For this review, take the finished solid that the model builds, in its own axes (mm). A direction names the side the tool comes from. Round coordinates to 2 decimals unless told otherwise and drop trailing zeros. Order: outer loops, then holes, each group sorted by start corner. A loop starts at its lowest first (then second) coordinate and runs counter-clockwise, first axis right, second up.
from build123d import *

# Parameters (mm, degrees)
EXTRUDE_1_DEPTH     = 28
SKETCH_2_W          = 5
SKETCH_2_H          = 20
CUT_EXTRUDE_1_DEPTH = 5
SKETCH_3_R          = 1.5
CUT_EXTRUDE_2_DEPTH = 118.553755913


with BuildPart() as part:
    # 草圖1 → 填料-伸長1 (new body)
    with BuildSketch(Plane.XY):
        Polygon((-17.451364004, -6.196122823), (-17.451364004, -11.196122823), (-22.451364004, -11.196122823), (-22.451364004, 105.303877177), (-17.451364004, 105.303877177), (-17.451364004, 100.303877177), (24.548635996, 100.303877177), (24.548635996, 95.303877177), (-17.451364004, 95.303877177), (-17.451364004, -1.196122823), (16.048635996, -1.196122823), (16.048635996, -6.196122823), align=None)
    extrude(amount=EXTRUDE_1_DEPTH)

    # 草圖2 → 除料-伸長1 (cut)
    with BuildSketch(Plane(origin=(0, 0, 0), x_dir=(-1, 0, 0), z_dir=(0, 0, -1))):
        with Locations((19.951364004, 47.053877177)):
            Rectangle(SKETCH_2_W, SKETCH_2_H)
    extrude(amount=-CUT_EXTRUDE_1_DEPTH, mode=Mode.SUBTRACT)

    # 草圖3 → 除料-伸長2 (cut, through all)
    with BuildSketch(Plane.XZ.offset(6.196122823)):
        with Locations(Location((-2.451364004, 15, 0), (0, 0, 270))):
            Circle(SKETCH_3_R)
    extrude(amount=-CUT_EXTRUDE_2_DEPTH, mode=Mode.SUBTRACT)


solid = part.part
(1) Wall thickness on L1, parallel to Y at x = 14.5, z = 8; L2, parallel to X at y = -3.45, z = 15; L3, parallel to X at y = 22, z = 25: over which ranges is each line inside the solid? List them lowest first.
(2) Add section A-A on x = -8.5. Give the boundary of the cut face in (y, z).
(3) Add section D-D on y = 12.5. Give the boundary of the cut face in (x, z).
(4) Add section B-B on z = 15. Give the boundary of the cut face in (x, y), plus the area to 3 significant figures.
(5) Add section C-C on y = 50. Give the boundary of the cut face in (x, z).
(6) Tool access review of faces 4 (the face through (-19, 6, 0)), 5 (the face through (4, 95.304, 14)), 6 (the face through (-17.451, -9, 14)), 7 (the face through (-20, 47, 5)), 8 (the face through (-17.451, 103, 14)): name each direction out of +Z, -Z, +X, -X, +Y, -Y from which nothing blocks a thin tool from reaching the whole face with its end or side.
(7) Draft analysis for pull direction Y (two halves, no side actions). For faces 1 (the face through (0, -6.196, 14)), 2 (the face through (24.549, 98, 14)), 3 (the face through (-20, 37.054, 2)), state which applies: pulls with the +Y half, pulls with the -Y half, needs draft (parallel to the pull), parting line crosses it, or undercut.
(8) Clearance check with flat-ended pins moving along their axes: P1, Ø8.5, axis at x = -2, z = 15.5, coming from the +Y side; P2, Ø2, axis at y = 36, z = 14.5, coming from the +X side; P3, Ø14, axis at x = -1, z = 16.5, coming from the -Y side. State where each tip first meets the part, or that it passes through.
Here are the results:
1. L1: y = -6.2 to -1.2, 95.3 to 100.3
1. L2: x = -22.45 to -3.95, -0.95 to 16.05
1. L3: x = -22.45 to -17.45
2. outline: (-6.2, 0) - (-1.2, 0) - (-1.2, 28) - (-6.2, 28) - close; (95.3, 0) - (100.3, 0) - (100.3, 28) - (95.3, 28) - close
3. outline: (-22.45, 0) - (-17.45, 0) - (-17.45, 28) - (-22.45, 28) - close
4. outline: (-22.45, -11.2) - (-17.45, -11.2) - (-17.45, -6.2) - (-3.95, -6.2) - (-3.95, -1.2) - (-17.45, -1.2) - (-17.45, 95.3) - (-3.95, 95.3) - (-3.95, 100.3) - (-17.45, 100.3) - (-17.45, 105.3) - (-22.45, 105.3) - close; (-0.95, -6.2) - (16.05, -6.2) - (16.05, -1.2) - (-0.95, -1.2) - close; (-0.95, 95.3) - (24.55, 95.3) - (24.55, 100.3) - (-0.95, 100.3) - close
4. area: 930 mm2
5. outline: (-22.45, 5) - (-17.45, 5) - (-17.45, 28) - (-22.45, 28) - close
6. face 4: -Z, +X, -X, +Y, -Y
6. face 5: +Z, -Z, +X
6. face 6: +Z, -Z, +X, -Y
6. face 7: -Z, +X, -X
6. face 8: +Z, -Z, +X, +Y
7. face 1: pulls with the -Y half
7. face 2: needs draft
7. face 3: undercut
8. P1: stops at y = 100.3
8. P2: stops at x = -17.45
8. P3: stops at y = -6.2
